Source: three-view drawing plus pictorial views. Frame: mm from the lowest corner of the part. A direction names the side the tool comes from. Coordinates: 2 decimals unless noted, no trailing zeros. Order: outer loops, then holes, each group sorted by start corner. A loop starts at its lowest first (then second) coordinate and runs counter-clockwise, first axis right, second up. Notation, with made-up numbers: (70, 62.5) - (93, 62.5) arc R17 cw to (93, 76.5) - close; hole circle Ø8 at (-8, 2). An arc over 180 degrees is marked (long way). One line per question, with ' | ' between items.
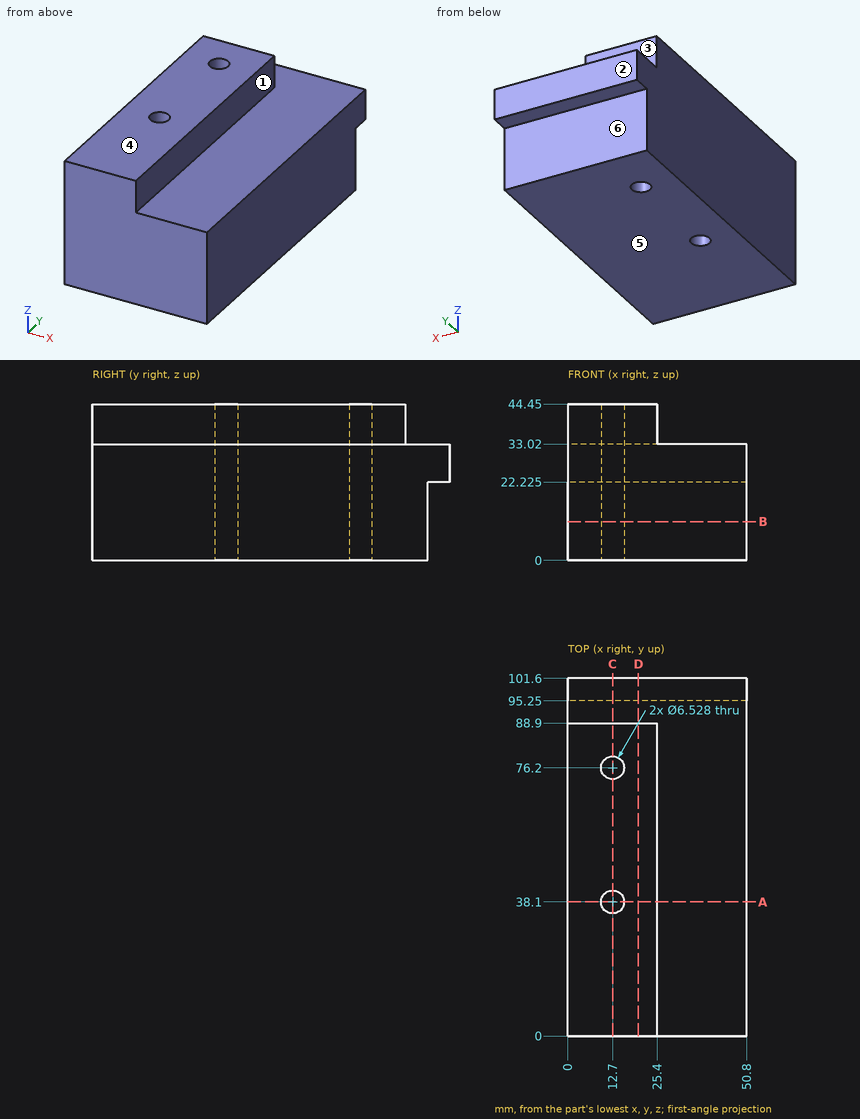
(1) Material intervals for L1, parallel to Y at x = 12.7, z = 28.5; L2, parallel to Y at x = 12.7, z = 13; L3, parallel to X at y = 38, z = 20, sorted ascending. Write a range as from..to.
Taken from the geometry:
L1: y = 0..34.84, 41.36..72.94, 79.46..101.6 | L2: y = 0..34.84, 41.36..72.94, 79.46..95.25 | L3: x = 0..9.44, 15.96..50.8
(2) Cut plane A-A (y = 38.1). Return the cut outline in (x, z), and give its area (3 significant figures).
Taken from the geometry:
outline: (0, 0) - (9.44, 0) - (9.44, 44.45) - (0, 44.45) - close; (15.96, 0) - (50.8, 0) - (50.8, 33.02) - (25.4, 33.02) - (25.4, 44.45) - (15.96, 44.45) - close | area: 1,680 mm²
(3) Pin query (flat end, axial travel): P1, Ø6.5, axis at x = 24, z = 15, coming from the +Y side; P2, Ø1.9, axis at x = 18.5, y = 97, coming from the -Z side (3 decimals); P3, Ø9, axis at x = 11.5, z = 40, coming from the +Y side. Return the tip coordinate at first contact, or that it passes through.
Taken from the geometry:
P1: stops at y = 95.25 | P2: stops at z = 22.225 | P3: stops at y = 88.9
(4) Pull-direction query (Z, two-part tool) for the marked faces 4, 5 and 6; classes: pulls with the +Z half, pulls with the -Z half, needs draft (parallel to the pull), parting line crosses it, or undercut.
Taken from the geometry:
face 4: pulls with the +Z half | face 5: pulls with the -Z half | face 6: needs draft
(5) Set-up query: the marked faces 1, 2 and 3. Return all of +Z, -Z, +X, -X, +Y, -Y with unobstructed straight access to the full face (end or side cutting, diameter ignored); none if empty.
Taken from the geometry:
face 1: +Z, +X, +Y, -Y | face 2: +Z, -Z, +X, -X, +Y | face 3: +Z, +X, -X, +Y
(6) Cut plane B-B (z = 11). Return the cut outline in (x, y), and give its area (3 significant figures).
Taken from the geometry:
outline: (0, 0) - (50.8, 0) - (50.8, 95.25) - (0, 95.25) - close; hole circle Ø6.53 at (12.7, 38.1); hole circle Ø6.53 at (12.7, 76.2) | area: 4,770 mm²
(7) Cut plane D-D (x = 20). Return the cut outline in (y, z) (3 decimals).
Taken from the geometry:
outline: (0, 0) - (95.25, 0) - (95.25, 22.225) - (101.6, 22.225) - (101.6, 33.02) - (88.9, 33.02) - (88.9, 44.45) - (0, 44.45) - close
(8) Cut plane C-C (x = 12.7). State how many separate pieces and enclosed holes the cut face has, and give its area (3 significant figures).
Taken from the geometry:
separate pieces: 3 | enclosed holes: 0 | area: 3,650 mm²
